from build123d import *

# Parameters (mm, degrees)
F0_R     = 5.677699
F1_DEPTH = 6.35


with BuildPart() as f1:
    # F0 (on Front) → F1 (new body)
    with BuildSketch(Plane.XZ):
        with Locations((-3.173587, 2.108483)):
            Circle(F0_R)
        Polygon((-5.57913, 0), (-5.57913, 3.175), (-2.789565, 4.691229), (0, 3.175), (0, 0), (-2.789565, -1.516229), align=None, mode=Mode.SUBTRACT)
    extrude(amount=F1_DEPTH)


solid = f1.part
Here's how the part is built. I have some questions about the finished solid (model axes, mm). A direction names the side the tool comes from. Round coordinates to 2 decimals unless told otherwise and drop trailing zeros. Write each loop counter-clockwise with the first axis right and the second up, starting at its lowest first coordinate (ties: lowest second). Pieces come first, ordered by that corner, then holes. Notation, with made-up numbers: (77, -32.75) -> (121, -32.75) arc R5 cw to (121, -27.75) -> close; hole circle Ø10 at (42.5, -8.5). An arc over 180 degrees is marked (long way). One line per item, written item: value.
1) If I drill on line 1 (Z direction, x = -0.5, y = -5.5); line 2 (Z direction, x = -3, y = -2.5); line 3 (X direction, y = -4, z = 0.5), over which ranges is the centre line in solid material (lowest first)? Write a range as [from, to].
Filled sheet:
line 1: z = [-2.9, -0.27], [3.45, 7.12]
line 2: z = [-3.57, -1.4], [4.58, 7.78]
line 3: x = [-8.62, -5.58], [0, 2.27]
2) For faces 5 (the face through (-4.16, -3.13, -0.77)), 6 (the face through (-6, -6.35, 2)), which set-ups out of +Z, -Z, +X, -X, +Y, -Y let a thin tool reach every point of the face, with its end or its side?
Filled sheet:
face 5: +Y, -Y
face 6: +Z, -Z, +X, -X, -Y
3) Suppose I cut it at D-D on x = -1. List the corners of the cut face in (y, z) for me, plus the area to 3 significant figures.
Filled sheet:
outline: (-6.35, -3.14) -> (0, -3.14) -> (0, -0.54) -> (-6.35, -0.54) -> close; (-6.35, 3.72) -> (0, 3.72) -> (0, 7.35) -> (-6.35, 7.35) -> close
area: 39.5 mm2
4) Suppose I cut it at A-A on x = -4.5. List the corners of the cut face in (y, z) for me.
Filled sheet:
outline: (-6.35, -3.41) -> (0, -3.41) -> (0, -0.59) -> (-6.35, -0.59) -> close; (-6.35, 3.76) -> (0, 3.76) -> (0, 7.63) -> (-6.35, 7.63) -> close
5) We'd pull the mould along X, two halves only. Please class faces 1 (the face through (-4.404, -3.131, -3.434)), 2 (the face through (-1.38, -3.13, -0.75)), 3 (the face through (0, -3, 2)), 4 (the face through (-6, 0, 2)): released by +X, released by -X, zero draft, split by the parting line, or undercut.
Filled sheet:
face 1: split by the parting line
face 2: undercut
face 3: undercut
face 4: zero draft
6) Suppose I cut it at C-C on z = -2. List the corners of the cut face in (x, y) for me, plus the area to 3 significant figures.
Filled sheet:
outline: (-7.09, -6.35) -> (0.75, -6.35) -> (0.75, 0) -> (-7.09, 0) -> close
area: 49.8 mm2
7) Suppose I cut it at B-B on y = -3.75. List the corners of the cut face in (x, z) for me (3 decimals), plus the area to 3 significant figures.
Filled sheet:
outline: circle Ø11.355 at (-3.174, 2.108); hole (-5.579, 0) -> (-2.79, -1.516) -> (0, 0) -> (0, 3.175) -> (-2.79, 4.691) -> (-5.579, 3.175) -> close
area: 75.1 mm2
8) I'm going to push flat-ended pins straight in: pin 1 Ø1.5 at (y, z) = (-5, -1) entering from -X; pin 2 Ø2 at (y, z) = (-3.5, -2) entering from -X; pin 3 Ø1.5 at (x, y) = (-6.5, -5) entering from +Z. Where does each tip first touch, or does it pass through?
Filled sheet:
pin 1: stops at x = -8.34
pin 2: stops at x = -7.92
pin 3: stops at z = 7.17
